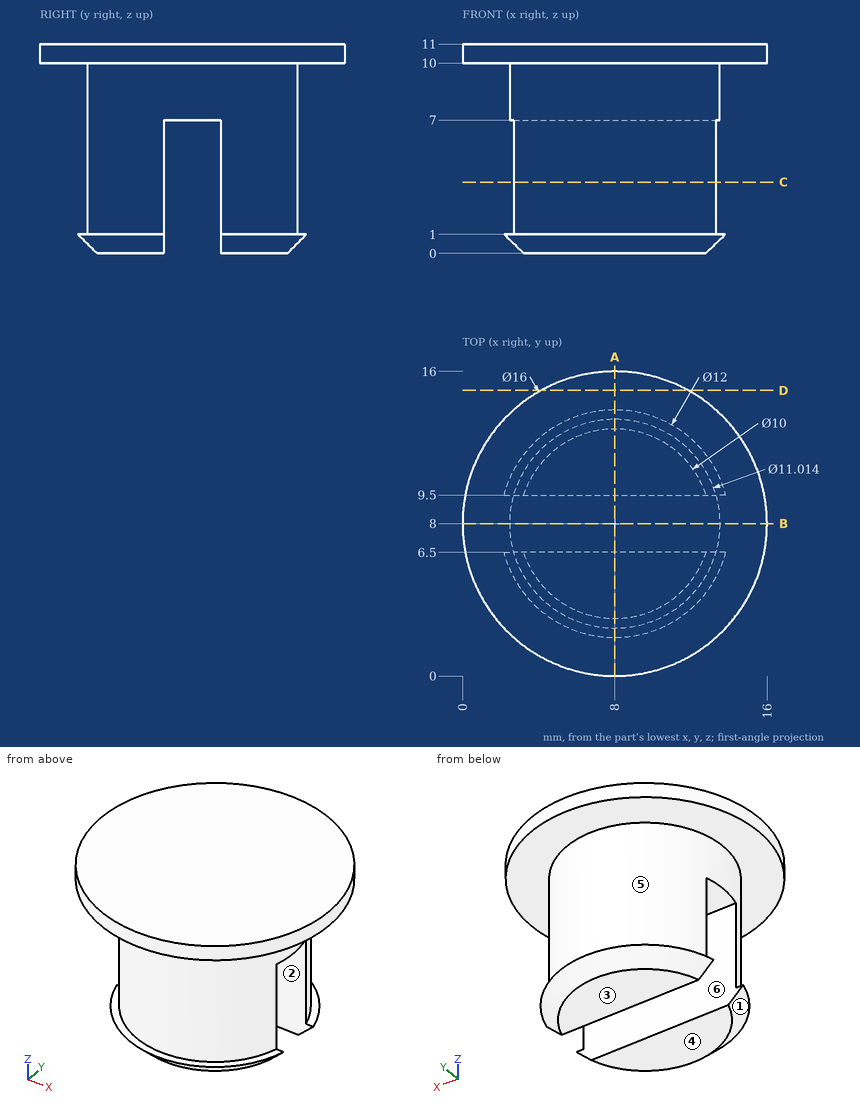
Design review of the part shown in the three views and the two pictorial views. Dimensions are in mm from the part's minimum x, y and z. A direction names the side the tool comes from. Give positions to 0.01 mm unless a question says otherwise; leave off trailing zeros. Loops run counter-clockwise (first coordinate to the right, second up) from the corner with the lowest first, then second, coordinate; pieces in that order, holes last. Notation, with made-up numbers: M 75.5,7.5 L 116.5,7.5 A25 cw 116.5,26.5 Z; hole C 86.5,-8.75 d4. An arc over 180 degrees is marked long. Write item = value, one per line.
Q1. We need section C-C (z = 3.75). Give the boundary of the cut face in (x, y).
Output values:
outline = M 2.7,6.5 A5.51 ccw 13.3,6.5 Z; M 2.7,9.5 L 13.3,9.5 A5.51 ccw Z
Q2. We need section A-A (x = 8). Give the boundary of the cut face in (y, z).
Output values:
outline = M 0,10 L 2.49,10 L 2.49,1 L 2,1 L 3,0 L 6.5,0 L 6.5,7 L 9.5,7 L 9.5,0 L 13,0 L 14,1 L 13.51,1 L 13.51,10 L 16,10 L 16,11 L 0,11 Z
Q3. For the marked faces 4, 5 and 6, list the 3-axis set-ups (+Z, -Z, +X, -X, +Y, -Y) from which the entire face can be reached by the end or side of a thin tool; tool diameter is ignored.
Output values:
face_4 = -Z, +X, -X, +Y, -Y
face_5 = none
face_6 = -Z, +X, -X
Q4. Insertion check: pin 1 (1 mm diameter, centred on y = 4, z = 5, fed in from +X); pin 2 (3 mm diameter, centred on y = 13, z = 6, fed in from -X); pin 3 (1.5 mm diameter, centred on x = 6, y = 8, fed in from -Z). Each pin has a flat end and moves straight along its axis. Give the tip position at first contact, or say it passes through.
Output values:
pin_1 = 12.25
pin_2 = 3.75
pin_3 = 7
Q5. To check wall thickness, follow line 1 (Z direction, x = 7.75, y = 14.75); line 2 (Z direction, x = 10, y = 7.25); line 3 (Y direction, x = 11.75, z = 5.5). State the ranges of each line that lie inside material, in increasing order. Write a range as [from, to].
Output values:
line_1 = [10, 11]
line_2 = [7, 11]
line_3 = [3.97, 6.5], [9.5, 12.03]
Q6. We need section D-D (y = 15). Give the boundary of the cut face in (x, z), plus the area to 3 significant figures.
Output values:
outline = M 4.13,10 L 11.87,10 L 11.87,11 L 4.13,11 Z
area = 7.75 mm^2
Q7. We need section B-B (y = 8). Give the boundary of the cut face in (x, z).
Output values:
outline = M 0,10 L 2.49,10 L 2.49,7 L 13.51,7 L 13.51,10 L 16,10 L 16,11 L 0,11 Z
Q8. Draft analysis for pull direction Y (two halves, no side actions). For the marked faces 1, 2 and 3, state which applies: +Y half, -Y half, draft (parallel to the pull), parting line (faces both ways), or undercut.
Output values:
face_1 = -Y half
face_2 = undercut
face_3 = draft
